Autodesk Inventor part; units mm, degrees
ref_plane "YZ Plane" through (0, 0, 0) normal (1, 0, 0) x (0, 1, 0)
ref_plane "XZ Plane" through (0, 0, 0) normal (0, 1, 0) x (-1, 0, 0)
ref_plane "XY Plane" through (0, 0, 0) normal (0, 0, 1) x (1, 0, 0)
sketch "Эскиз1" plane through (0, 0, 0) normal (0, 1, 0) x (-1, 0, 0)
  line L0 (4, 13) -> (-1, 13)
  line L1 (-5, 9) -> (-5, -27)
  line L2 (-1, -31) -> (4, -31)
  line L3 (8, -27) -> (8, 9)
  circle A0 centre (1.5, 7) radius 2
  circle A1 centre (1.5, -25) radius 2
  arc A2 (8, 9) -> (4, 13) centre (4, 9) ccw
  arc A3 (-1, 13) -> (-5, 9) centre (-1, 9) ccw
  arc A4 (-5, -27) -> (-1, -31) centre (-1, -27) ccw
  arc A5 (4, -31) -> (8, -27) centre (4, -27) ccw
  point P0 (0, 0)
  point P1 (-5, -31)
  point P2 (-5, 13)
  point P3 (8, -31)
  dimension "d0" = 13
  dimension "d1" = 44
  dimension "d2" = 4
  dimension "d3" = 4
  dimension "d4" = 32
  dimension "d5" = 6.5
  dimension "d6" = 6
  dimension "d7" = 4
extrude "Выдавливание1" add sketch "Эскиз1" along normal blind 35
sketch "Эскиз2" plane through (-8, 0, -27) normal (-1, 0, 0) x (0, 0, 1)
  circle A0 centre (18, 15) radius 10.1
  circle A1 centre (18, 15) radius 5.05
  line L0 (0, 0) -> (36, 0)
  line L1 (36, 0) -> (36, 35)
  circle A2 centre (18, 15) radius 7.5 construction
  circle A3 centre (18, 22.5) radius 1.5
  line L2 (18, 15) -> (25.5, 15)
  line L3 (18, 15) -> (24.4952, 11.25)
  line L4 (18, 15) -> (25.5, 15) construction
  circle A4 centre (24.4952, 11.25) radius 1.5
  line L5 (18, 15) -> (10.5, 15)
  line L6 (18, 15) -> (24.4952, 11.25)
  line L7 (18, 15) -> (25.5, 15) construction
  line L8 (18, 15) -> (11.5048, 11.25)
  line L9 (18, 15) -> (25.5, 15) construction
  circle A5 centre (11.5048, 11.25) radius 1.5
  point P0 (27, 0)
  dimension "d10" = 20.2
  dimension "d11" = 10.1
  dimension "d12" = 15
  dimension "d13" = 18
  dimension "d14" = 15
  dimension "d15" = 3
  dimension "d16" = 30
  dimension "d17" = 3
  dimension "d18" = 30
  dimension "d19" = 150
  dimension "d20" = 3
extrude "Выдавливание2" cut sketch "Эскиз2" against normal blind 40 contours L2 L5 A1 | A1 L3 L2 | L5 L8 A1 | A1 L8 L3 | A3 | A4 | A5
sketch "Эскиз3" plane through (-8, 0, -27) normal (-1, 0, 0) x (0, 0, 1)
  circle A0 centre (18, 15) radius 5
  circle A1 centre (18, 15) radius 10.1
  line L0 (0, 0) -> (36, 0)
  point P0 (27, 0)
  dimension "d23" = 20.2
  dimension "d29" = 15
extrude "Выдавливание3" cut sketch "Эскиз3" against normal blind 10
chamfer "Фаска1" distance 0.5 angle 45 16 edges at (-8, 35, -9) (-6.8284, 35, 11.8284) (-1.5, 35, 13) (3.8284, 35, 11.8284) (5, 35, -9) (3.8284, 35, -29.8284) (-1.5, 35, -31) (-6.8284, 35, -29.8284) (-8, 0, -9) (-6.8284, 0, 11.8284) (-1.5, 0, 13) (3.8284, 0, 11.8284) (5, 0, -9) (3.8284, 0, -29.8284) (-1.5, 0, -31) (-6.8284, 0, -29.8284)
fillet "Сопряжение1" radius 2 3 edges at (5, 22.5, -10.5) (5, 11.25, -4.0048) (5, 11.25, -16.9952)
properties part number "fastenin_motor"
The listing builds one solid part. Answer for the finished solid, in the listing's coordinates (mm). Coordinates: 2 decimals unless noted, no trailing zeros. Write each loop counter-clockwise with the first axis right and the second up, starting at its lowest first coordinate (ties: lowest second). Pieces come first, ordered by that corner, then holes. Notation, with made-up numbers: M -24.75,47.5 L 5.25,47.5 A3 ccw 5.25,51.5 Z; hole C -5.5,85.5 d1. An arc over 180 degrees is marked long. Use a Markdown table: item, result. Add a question column.
1. Straight lines are drawn through the part: line 1 along Y through (x, z) = (2.6, -9); line 2 along Z through (x, y) = (-1.5, 19); line 3 along Z through (x, y) = (-2, 23.5). For each, find the intervals that lie inside material, in ascending order. Write a range as [from, to].
2. Section B-B (y = 30) is taken. Give the vertices of the cut face in (x, z).
3. Section D-D (z = -9) is taken. Give the vertices of the cut face in (x, y), plus the area to 3 significant figures.
4. Section C-C (z = -25) is taken. Give the vertices of the cut face in (x, y), plus the area to 4 significant figures.
5. Given P1, Ø5, axis at y = 11.25, z = -15.5, coming from the -X side; P2, Ø4, axis at y = 22.5, z = -9, coming from the +X side, each flat-ended and moving along its own axis, determine where each tip first touches the part or whether it passes through.
6. For a pull along X with two mould halves and no side action, classify faces 1 (the cylindrical face through (-3.07, 25.014, -10.315)), 2 (the cylindrical face through (-3.408, 17.255, 6.399)), 3 (the flat face through (-8, 25, -13)) as +X half, -X half, draft (parallel to the pull), parting line (faces both ways), or undercut.
7. Section A-A (x = -1.5) is taken. Give the vertices of the cut face in (y, z), plus the area to 3 significant figures.
Data:
| question | item | result |
|---|---|---|
| 1 | line 1 | y = [0, 9.95], [20.05, 21], [24, 35] |
| 1 | line 2 | z = [-31, -27], [-23, -18.27], [0.27, 5], [9, 13] |
| 1 | line 3 | z = [-31, -26.94], [-23.06, -14.46], [-3.54, 5.06], [8.94, 13] |
| 2 | outline | M -8,-27 A4 ccw -4,-31 L 1,-31 A4 ccw 5,-27 L 5,9 A4 ccw 1,13 L -4,13 A4 ccw -8,9 Z; hole C -1.5,-25 d4; hole C -1.5,7 d4 |
| 3 | outline | M -8,0.5 L -7.5,0 L 4.5,0 L 5,0.5 L 5,9.95 L 2,9.95 L 2,4.9 L -8,4.9 Z; M -8,25.1 L 2,25.1 L 2,24 L 3,24 A2 ccw 5,26 L 5,34.5 L 4.5,35 L -7.5,35 L -8,34.5 Z; M 2,20.05 L 4.7,20.05 A2 ccw 3,21 L 2,21 Z |
| 3 | area | 212 mm2 |
| 4 | outline | M -8,0.5 L -7.5,0 L -3.5,0 L -3.5,35 L -7.5,35 L -8,34.5 Z; M 0.5,0 L 4.5,0 L 5,0.5 L 5,34.5 L 4.5,35 L 0.5,35 Z |
| 4 | area | 314.5 mm2 |
| 5 | P1 | stops at x = 2 |
| 5 | P2 | stops at x = 4.32 |
| 6 | face 1 | draft |
| 6 | face 2 | undercut |
| 6 | face 3 | -X half |
| 7 | outline | M 0,-30.5 L 0.5,-31 L 34.5,-31 L 35,-30.5 L 35,-27 L 0,-27 Z; M 0,-23 L 35,-23 L 35,5 L 0,5 Z; M 0,9 L 35,9 L 35,12.5 L 34.5,13 L 0.5,13 L 0,12.5 Z; hole C 15,-9 d20.2 |
| 7 | area | 939 mm2 |
